Geometry: final body of the model. Coordinates: model frame, mm. A direction names the side the tool comes from. Round coordinates to 2 decimals unless told otherwise and drop trailing zeros. Loops run counter-clockwise (first coordinate to the right, second up) from the corner with the lowest first, then second, coordinate; pieces in that order, holes last. Notation, with made-up numbers: M -35,20.25 L 9,20.25 A18 cw 9,54.25 Z; hole C 88.25,31 d6. An arc over 180 degrees is marked long. Write each question's results on one line, items separated by ' | '.
```python
from build123d import *

# Parameters (mm, degrees)
EXTRUDE_590_DEPTH   = 29.6
EXTRUDE_638_DEPTH   = 9.5
FILLET_1_R          = 3
HOLE_WIZARD_M5_1_D  = 5.3
CUT_EXTRUDE_1_DEPTH = 5
CUT_EXTRUDE_2_DEPTH = 0.1


with BuildPart() as part:
    # 草图1 → Extrude 590 (new body)
    with BuildSketch(Plane(origin=(0, 0, 0), x_dir=(1, 0, 0), z_dir=(0, 1, 0))):
        with BuildLine():
            Line((4.608867317, -165), (-4.608867317, -165))
            Line((-4.608867317, -165), (-5.444719551, -194.923972433))
            ThreePointArc((-5.444719551, -194.923972433), (0, -195), (5.444719551, -194.923972433))
            Line((5.444719551, -194.923972433), (4.608867317, -165))
        make_face()
    extrude(amount=EXTRUDE_590_DEPTH)

    # 草图1<3> → Extrude 638 (add)
    with BuildSketch(Plane(origin=(0, 0, 0), x_dir=(1, 0, 0), z_dir=(0, 1, 0))):
        with BuildLine():
            ThreePointArc((5.444719551, -194.923972433), (0, -195), (-5.444719551, -194.923972433))
            Line((-5.444719551, -194.923972433), (-5.584327745, -199.922023008))
            ThreePointArc((-5.584327745, -199.922023008), (0, -200), (5.584327745, -199.922023008))
            Line((5.584327745, -199.922023008), (5.444719551, -194.923972433))
        make_face()
    extrude(amount=EXTRUDE_638_DEPTH)

    # 圆角1
    fillet_1_edges = [part.edges().sort_by_distance(p)[0] for p in [
        (0, 0, 165),
        (-4.608867317, 14.8, 165),
        (4.608867317, 14.8, 165),
    ]]
    fillet(fillet_1_edges, radius=FILLET_1_R)

    # M5 间隙孔1 (through all)
    with Locations(Plane(origin=(0, 29.6, 0), x_dir=(1, 0, 0), z_dir=(0, 1, 0))):
        with Locations((0, -187), (0, -175)):
            Hole(HOLE_WIZARD_M5_1_D / 2)

    # 草图6 → 切除-拉伸1 (cut)
    with BuildSketch(Plane.XZ):
        Polygon((0, 179.792007234), (-4.15, 177.396003617), (-4.15, 172.603996383), (0, 170.207992766), (4.15, 172.603996383), (4.15, 177.396003617), align=None)
        Polygon((0, 191.792007234), (-4.15, 189.396003617), (-4.15, 184.603996383), (0, 182.207992766), (4.15, 184.603996383), (4.15, 189.396003617), align=None)
    extrude(amount=-CUT_EXTRUDE_1_DEPTH, mode=Mode.SUBTRACT)

    # 草图7 → 切除-拉伸2 (cut)
    with BuildSketch(Plane(origin=(0, 0, 0), x_dir=(-0.02792163872356911, 0, -0.9996101150403545), z_dir=(0.9996101150403545, 0, -0.02792163872356911))):
        with BuildLine():
            Line((-172.3983953, 27.023076923), (-172.712497864, 27.023076923))
            add(Edge.make_bspline(
                [(-172.712497864, 27.023076923), (-172.710450711, 27.064747811), (-172.706430157, 27.146588325), (-172.687601868, 27.265912232), (-172.660660991, 27.379967031), (-172.622569537, 27.487836945), (-172.575263259, 27.590475752), (-172.518533231, 27.687475767), (-172.451339381, 27.778466956), (-172.375132647, 27.862605799), (-172.292364008, 27.93979337), (-172.203058068, 28.006448613), (-172.109213041, 28.062766284), (-172.011113642, 28.109847526), (-171.907653079, 28.145187372), (-171.799770221, 28.171409012), (-171.686991084, 28.187185357), (-171.610151062, 28.188881143), (-171.571071582, 28.18974359)],
                knots=[0, 0, 0, 0, 1.10065271, 2.161652631, 3.183658789, 4.190468796, 5.17591951, 6.163126047, 7.15150782, 8.156236427, 9.156009102, 10.134482811, 11.092018607, 12.041330605, 13.001268258, 13.972401359, 14.968799086, 16, 16, 16, 16], degree=3))
            add(Edge.make_bspline(
                [(-171.571071582, 28.18974359), (-171.532693508, 28.188845133), (-171.457281963, 28.187079698), (-171.347219949, 28.171918669), (-171.242442654, 28.148173078), (-171.143154888, 28.114857661), (-171.050148823, 28.070073234), (-170.962725779, 28.016275695), (-170.879844968, 27.954055864), (-170.805238184, 27.88080205), (-170.736730105, 27.802599666), (-170.67762785, 27.719111762), (-170.627014686, 27.632882477), (-170.584827007, 27.543254275), (-170.553770868, 27.449383247), (-170.53019266, 27.352636044), (-170.516865246, 27.252011233), (-170.514819822, 27.183904677), (-170.513779915, 27.149278846)],
                knots=[0, 0, 0, 0, 1.111607364, 2.184268762, 3.212621178, 4.221274766, 5.211760367, 6.196651075, 7.1921475, 8.207485113, 9.220403448, 10.201281604, 11.166441695, 12.114753415, 13.065576456, 14.026450734, 14.996634279, 16, 16, 16, 16], degree=3))
            add(Edge.make_bspline(
                [(-170.513779915, 27.149278846), (-170.515473178, 27.100531012), (-170.51882999, 27.003890798), (-170.547544366, 26.861875935), (-170.592390877, 26.724282516), (-170.646388234, 26.613545214), (-170.700860678, 26.52431172), (-170.749948186, 26.450843015), (-170.807412997, 26.371737547), (-170.874091495, 26.28726021), (-170.948604367, 26.196749304), (-171.03162653, 26.100259509), (-171.123750012, 25.998787739), (-171.188408513, 25.929482138), (-171.221912928, 25.893569712)],
                knots=[0, 0, 0, 0, 1.184426356, 2.348067706, 3.509069118, 4.696110526, 5.333549288, 6.050745305, 6.844228056, 7.710549037, 8.667450064, 9.695053472, 10.805634456, 12, 12, 12, 12], degree=3))
            Line((-171.221912928, 25.893569712), (-172.09761405, 24.958974359))
            Line((-172.09761405, 24.958974359), (-170.46890812, 24.958974359))
            Line((-170.46890812, 24.958974359), (-170.46890812, 24.6))
            Line((-170.46890812, 24.6), (-172.847113249, 24.6))
            Line((-172.847113249, 24.6), (-171.489741454, 26.048517628))
            add(Edge.make_bspline(
                [(-171.489741454, 26.048517628), (-171.456693567, 26.083015935), (-171.39321534, 26.149280121), (-171.303432763, 26.246023081), (-171.222793775, 26.335772622), (-171.150776382, 26.418359171), (-171.088942877, 26.494990738), (-171.034070645, 26.563185442), (-170.990105054, 26.625939892), (-170.942389658, 26.698680506), (-170.896175677, 26.787492823), (-170.856463321, 26.896026513), (-170.832248472, 27.007753765), (-170.829343637, 27.083255802), (-170.827882479, 27.121233974)],
                knots=[0, 0, 0, 0, 1.329631726, 2.553950428, 3.673215718, 4.687767853, 5.603093632, 6.413772471, 7.123043292, 7.734684054, 8.834405432, 9.900288307, 10.943827018, 12, 12, 12, 12], degree=3))
            add(Edge.make_bspline(
                [(-170.827882479, 27.121233974), (-170.828518222, 27.145115373), (-170.829771148, 27.192181023), (-170.840828845, 27.261186782), (-170.857539351, 27.327751596), (-170.881484609, 27.392080215), (-170.913091349, 27.453525867), (-170.951564729, 27.512163347), (-170.995954793, 27.568852313), (-171.047306062, 27.622005611), (-171.103717582, 27.670686816), (-171.163311832, 27.713810902), (-171.226361936, 27.749850012), (-171.292602058, 27.779393509), (-171.361847527, 27.802568891), (-171.434232273, 27.81862747), (-171.509556289, 27.828709954), (-171.560989784, 27.830074126), (-171.587197383, 27.830769231)],
                knots=[0, 0, 0, 0, 0.991446411, 1.95395049, 2.89581595, 3.838931463, 4.798493298, 5.75982156, 6.748411868, 7.785213223, 8.824556874, 9.840280684, 10.836137867, 11.835679398, 12.848801643, 13.863922112, 14.911575587, 16, 16, 16, 16], degree=3))
            add(Edge.make_bspline(
                [(-171.587197383, 27.830769231), (-171.614568216, 27.830054199), (-171.668320012, 27.828649993), (-171.747239045, 27.818827329), (-171.822524823, 27.801881489), (-171.894366726, 27.778704814), (-171.962886312, 27.749246266), (-172.027750356, 27.712554521), (-172.088813245, 27.668771028), (-172.146189768, 27.619130471), (-172.199053747, 27.56386287), (-172.245500623, 27.502252907), (-172.286084637, 27.435425492), (-172.321493871, 27.363560941), (-172.350249561, 27.286007161), (-172.372222711, 27.203039456), (-172.389609558, 27.115018075), (-172.395418079, 27.05423299), (-172.3983953, 27.023076923)],
                knots=[0, 0, 0, 0, 1.031018746, 2.02475058, 2.990194455, 3.934040569, 4.864654155, 5.795059489, 6.735614925, 7.690564532, 8.649604399, 9.611025574, 10.590972636, 11.591080095, 12.624614302, 13.701020113, 14.821632451, 16, 16, 16, 16], degree=3))
        make_face()
    extrude(amount=-CUT_EXTRUDE_2_DEPTH, mode=Mode.SUBTRACT)


solid = part.part
```
1. Pin query (flat end, axial travel): P1, Ø1.5, axis at y = 15.5, z = 191, coming from the +X side; P2, Ø4, axis at x = 1, z = 173.5, coming from the -Y side; P3, Ø1.5, axis at x = -3.5, y = 5.5, coming from the +Z side; P4, Ø6, axis at x = 0, z = 187, coming from the +Y side. Return the tip coordinate at first contact, or that it passes through.
Answer key:
P1: stops at x = 5.36 | P2: stops at y = 5 | P3: stops at z = 199.98 | P4: stops at y = 29.6
2. Section D-D (z = 175). Output: boundary loops of the cut face in (x, y).
Answer key:
outline: M -4.89,0 L -4.15,0 L -4.15,5 L -2.65,5 L -2.65,29.6 L -4.89,29.6 Z; M 2.65,5 L 4.15,5 L 4.15,0 L 4.89,0 L 4.89,29.6 L 2.65,29.6 Z
3. Draft query along X for faces 1 (the face through (-2.1, 2.46, 171.42)), 2 (the face through (-0.07, 0.52, 166.31)). Return one class per face: pulls with the +X half, pulls with the -X half, needs draft (parallel to the pull), parting line crosses it, or undercut.
Answer key:
face 1: undercut | face 2: needs draft
4. Access query for faces 3 (the face through (4, 0, 184)), 4 (the face through (-2.1, 2.46, 183.42)), 5 (the face through (0, 5, 200)). Directions: +Z, -Z, +X, -X, +Y, -Y. A direction counts if a zero-diameter tool reaches every point of the face in a straight line with its end or side. Return the directions, or none.
Answer key:
face 3: +Z, -Z, +X, -X, -Y | face 4: -Y | face 5: +Z, +Y, -Y
5. Section B-B (x = 1.25). Output: boundary loops of the cut face in (y, z), then the cut area to 3 significant figures.
Answer key:
outline: M 0,168 A3 ccw 3,165 L 29.6,165 L 29.6,172.66 L 5,172.66 L 5,170.93 L 0,170.93 Z; M 0,179.07 L 5,179.07 L 5,177.34 L 29.6,177.34 L 29.6,184.66 L 5,184.66 L 5,182.93 L 0,182.93 Z; M 0,191.07 L 5,191.07 L 5,189.34 L 29.6,189.34 L 29.6,195 L 9.5,195 L 9.5,200 L 0,200 Z | area: 622 mm²
6. Ray query, probe 1 along Z at (x, y) = (0, 15.5); probe 2 along Z at (x, y) = (-1.75, 22); probe 3 along X at (y, z) = (13, 175). Return the intervals inside material, ascending.
Answer key:
probe 1: z = 165 to 172.35, 177.65 to 184.35, 189.65 to 195 | probe 2: z = 165 to 173.01, 176.99 to 185.01, 188.99 to 194.99 | probe 3: x = -4.89 to -2.65, 2.65 to 4.89
7. Section C-C (z = 187). Output: boundary loops of the cut face in (x, y).
Answer key:
outline: M -5.22,0 L -4.15,0 L -4.15,5 L -2.65,5 L -2.65,29.6 L -5.22,29.6 Z; M 2.65,5 L 4.15,5 L 4.15,0 L 5.22,0 L 5.22,29.6 L 2.65,29.6 Z
8. Section A-A (y = 13). Output: boundary loops of the cut face in (x, z), then the cut area to 3 significant figures.
Answer key:
outline: M -5.44,194.92 L -4.69,167.92 A3 ccw -1.69,165 L 1.69,165 A3 ccw 4.69,167.92 L 5.44,194.92 A195 ccw Z; hole C 0,175 d5.3; hole C 0,187 d5.3 | area: 254 mm²
